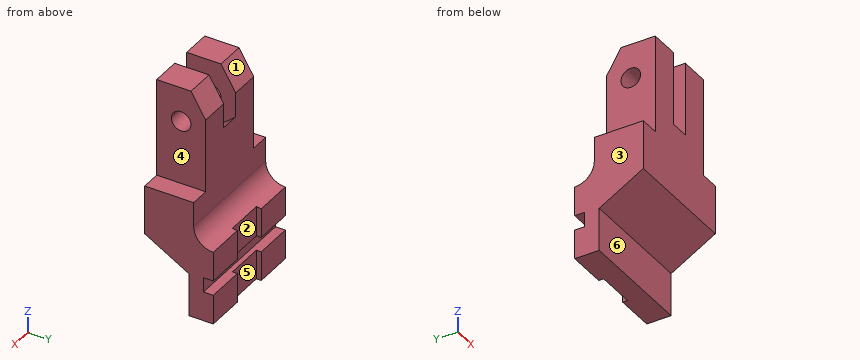
Autodesk Inventor part; units mm, degrees
ref_plane "XZ Plane" through (0, 0, 0) normal (0, 1, 0) x (-1, 0, 0)
ref_plane "XY Plane" through (0, 0, 0) normal (0, 0, 1) x (1, 0, 0)
sketch "Sketch1" plane through (0, 0, 0) normal (1, 0, 0) x (0, 1, 0)
  point P0 (0, 0)
sketch "Sketch2" plane through (0, 0, 0) normal (1, 0, 0) x (0, 1, 0)
  line L0 (70, -220) -> (0, -220) construction
  line L1 (0, -220) -> (0, 0) construction
  circle A0 centre (25, -35) radius 10
  line L2 (0, 0) -> (0, -150)
  line L3 (0, -150) -> (161.1976, -150) construction
  line L4 (70, -220) -> (45, -220)
  line L5 (70, -220) -> (70, -145)
  line L6 (70, -145) -> (70, -145)
  line L7 (50, -125) -> (50, 0) construction
  line L8 (50, 0) -> (0, 0) construction
  arc A1 (50, -125) -> (70, -145) centre (70, -125) ccw
  line L9 (50, -25) -> (35, 0)
  line L10 (0, -150) -> (116.4137, -150) construction
  line L11 (45, -220) -> (45, -175.9808)
  line L12 (50, -25) -> (50, -125)
  line L13 (35, 0) -> (0, 0)
  line L14 (0, -150) -> (45, -175.9808)
  line L15 (50, 0) -> (50, -50)
  line L16 (0, 0) -> (0, -75)
  circle A2 centre (-13.259, 14.018) radius 90 construction
  arc A3 (0, -75) -> (50, -50) centre (-13.259, 14.018) ccw
  line L17 (70, -190) -> (70, -175)
  line L18 (70, -175) -> (60, -175)
  line L19 (60, -175) -> (60, -190)
  line L20 (60, -190) -> (70, -190)
  point P0 (35, 0)
  point P1 (50, -145)
  point P2 (17.5, 0)
  dimension "d0" = 220
  dimension "d1" = 70
  dimension "d2" = 20
  dimension "d5" = 25
  dimension "d7" = 150
  dimension "d9" = 25
  dimension "d10" = 75
  dimension "d12" = 20
  dimension "d13" = 20
  dimension "d14" = 25
  dimension "d15" = 15
  dimension "d17" = 35
  dimension "d25" = 50
  dimension "d26" = 75
  dimension "d27" = 180
  dimension "d28" = 30
  dimension "d29" = 15
  dimension "d30" = 10
extrude "Extrusion1" add sketch "Sketch2" against normal blind 120
sketch "Sketch3" plane through (0, 70, -145) normal (0, 1, 0) x (1, 0, 0)
  line L0 (0, -145) -> (-120, -145)
  line L1 (-60, -145) -> (-60, 75)
  line L2 (0, 75) -> (-120, 75)
  line L3 (-120, -145) -> (-120, 75)
  line L4 (-120, 75) -> (0, 75)
  line L5 (0, -145) -> (-120, -145)
  line L6 (0, -145) -> (0, 75)
  line L7 (-100, -145) -> (-20, -145)
  line L8 (-20, -145) -> (-20, -45)
  line L9 (0, 30.9808) -> (-120, 30.9808)
  line L10 (-100, -145) -> (-100, -45)
  line L11 (-100, -45) -> (-120, -45)
  line L12 (-20, -45) -> (0, -45)
  dimension "d21" = 80
  dimension "d22" = 100
extrude "Extrusion2" cut sketch "Sketch3" against normal blind 120 contours L0 L8 L12 L6 | L0 L3 L11 L10
extrude "Extrusion3" cut sketch "Sketch2" against normal blind 120 contours L5 L20 L19 L18
ref_plane "Work Plane1" through (-60, 35, 0) normal (1, 0, 0) x (0, 1, 0)
sketch "Sketch4" plane through (-60, 35, 0) normal (1, 0, 0) x (0, 1, 0)
  line L0 (-35, 0) -> (0, 0)
  line L1 (-35, 0) -> (0, 0)
  line L2 (0, 0) -> (15, -25)
  line L3 (0, 0) -> (15, -25)
  line L4 (-35, 0) -> (-35, -75)
  arc A0 (-35, -75) -> (15, -50) centre (-48.259, 14.018) ccw
  line L5 (15, 0) -> (15, -50)
  line L6 (15, -25) -> (15, -100)
  line L7 (15, -50) -> (15, -100)
  line L8 (15, -100) -> (-35, -100)
  line L9 (-35, -100) -> (-35, -75)
  line L10 (15, 0) -> (-35, 0)
  dimension "d9" = 25
  dimension "d33" = 75
  dimension "d34" = 180
  dimension "d35" = 50
extrude "Extrusion4" cut sketch "Sketch4" along normal mid plane 20 contours L0 L2 L5 A0 L4
sketch "Sketch5" plane through (0, 45, -220) normal (0, 0, -1) x (-1, 0, 0)
  line L0 (0, 25) -> (120, 25)
  line L1 (60, 25) -> (60, -45) construction
  line L2 (40, 20) -> (80, 20)
  line L3 (40, 20) -> (40, 25)
  line L4 (80, 20) -> (80, 25)
  line L5 (40, 25) -> (80, 25)
  point P0 (0, -45)
  point P1 (60, 20)
  dimension "d38" = 40
  dimension "d39" = 5
extrude "Extrusion5" cut sketch "Sketch5" against normal blind 200
properties part number "thi1"
Source: CAD feature listing. Evaluate the final solid. Frame: model axes, mm. Face numbers are marked on the shaded views. A direction names the side the tool comes from. Give positions to 0.01 mm unless a question says otherwise; leave off trailing zeros. Loops run counter-clockwise (first coordinate to the right, second up) from the corner with the lowest first, then second, coordinate; pieces in that order, holes last. Notation, with made-up numbers: (-29, 47) -> (21, 47) arc R31 cw to (21, 74) -> close; hole circle Ø1 at (-2, 5.25). An arc over 180 degrees is marked (long way). Use a Markdown table: item, result. Add a question column.
(1) Pull-direction query (X, two-part tool) for the marked faces 1, 2 and 3; classes: +X half, -X half, draft (parallel to the pull), parting line (faces both ways), or undercut.
(2) Ray query, line 1 (X direction, y = 8.5, z = -49); line 2 (Y direction, x = -55.5, z = -118); line 3 (Y direction, x = -113, z = -179.5). Return the intervals inside material, ascending.
(3) Section query A-A (z = -35). Output: boundary loops of the cut face in (x, y).
(4) First-contact query: pin 1 Ø2 at (x, z) = (-91.5, -182.5) entering from -Y; pin 2 Ø5 at (x, z) = (-101.5, -116.5) entering from +Y; pin 3 Ø9 at (x, z) = (-61, -203.5) entering from +Y. Flat tips, straight axial feed; report the tip coordinate or a pass-through.
(5) Section query B-B (x = -87.5). Output: boundary loops of the cut face in (y, z), then the cut area to 3 significant figures.
(6) Section query C-C (y = 21.5). Output: boundary loops of the cut face in (x, z), then the cut area to 3 significant figures.
(7) Access query for the marked faces 4, 5 and 6. Directions: +Z, -Z, +X, -X, +Y, -Y. A direction counts if a zero-diameter tool reaches every point of the face in a straight line with its end or side. Return the directions, or none.
(8) Section query D-D (z = -201). Output: boundary loops of the cut face in (x, y), then the cut area to 3 significant figures.
Checked values:
| question | item | result |
|---|---|---|
| 1 | face 1 | draft |
| 1 | face 2 | undercut |
| 1 | face 3 | -X half |
| 2 | line 1 | -100 to -70, -50 to -20 |
| 2 | line 2 | 0 to 50 |
| 2 | line 3 | 45 to 60 |
| 3 | outline | (-100, 0) -> (-70, 0) -> (-70, 15) -> (-100, 15) -> close; (-100, 35) -> (-70, 35) -> (-70, 50) -> (-100, 50) -> close; (-50, 0) -> (-20, 0) -> (-20, 15) -> (-50, 15) -> close; (-50, 35) -> (-20, 35) -> (-20, 50) -> (-50, 50) -> close |
| 4 | pin 1 | y = 45 |
| 4 | pin 2 | y = 50 |
| 4 | pin 3 | y = 65 |
| 5 | outline | (0, -150) -> (45, -175.98) -> (45, -220) -> (70, -220) -> (70, -190) -> (60, -190) -> (60, -175) -> (70, -175) -> (70, -145) arc R20 cw to (50, -125) -> (50, -25) -> (35, 0) -> (0, 0) -> close; hole circle Ø20 at (25, -35) |
| 5 | area | 9,370 mm^2 |
| 6 | outline | (-120, -162.41) -> (0, -162.41) -> (0, -100) -> (-20, -100) -> (-20, -44.37) -> (-50, -44.37) -> (-50, -69) -> (-70, -69) -> (-70, -44.37) -> (-100, -44.37) -> (-100, -100) -> (-120, -100) -> close; (-100, -25.63) -> (-70, -25.63) -> (-70, 0) -> (-100, 0) -> close; (-50, -25.63) -> (-20, -25.63) -> (-20, 0) -> (-50, 0) -> close |
| 6 | area | 13,000 mm^2 |
| 7 | face 4 | +Z, +X, +Y, -Y |
| 7 | face 5 | +Z, -Z, +Y |
| 7 | face 6 | -Z, +X, -X, -Y |
| 8 | outline | (-120, 45) -> (0, 45) -> (0, 70) -> (-40, 70) -> (-40, 65) -> (-80, 65) -> (-80, 70) -> (-120, 70) -> close |
| 8 | area | 2,800 mm^2 |
